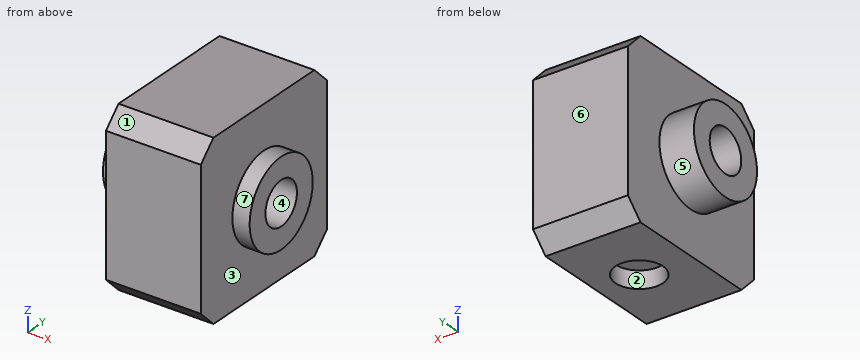
from build123d import *

# Parameters (mm, degrees)
SKETCH1_W           = 20
SKETCH1_H           = 20
BOSS_EXTRUDE1_DEPTH = 17
SKETCH2_R           = 15.353568197
SKETCH2_R_2         = 5
CUT_EXTRUDE1_DEPTH  = 2
CUT_EXTRUDE2_START  = -4
SKETCH3_R           = 15.635411304
SKETCH3_R_2         = 5
CUT_EXTRUDE2_DEPTH  = 4
SKETCH4_R           = 2.5
CUT_EXTRUDE3_DEPTH  = 23.113344387
CHAMFER1_SIZE       = 2
SKETCH5_R           = 2.75
CUT_EXTRUDE4_DEPTH  = 2


with BuildPart() as part:
    # Sketch1 → Boss-Extrude1 (new body)
    with BuildSketch(Plane(origin=(0, 0, 0), x_dir=(0, 0, -1), z_dir=(1, 0, 0))):
        Rectangle(SKETCH1_W, SKETCH1_H)
    extrude(amount=-BOSS_EXTRUDE1_DEPTH)

    # Sketch2 → Cut-Extrude1 (cut)
    with BuildSketch(Plane(origin=(0, 0, 0), x_dir=(0, 0, -1), z_dir=(1, 0, 0))):
        Circle(SKETCH2_R)
        Circle(SKETCH2_R_2, mode=Mode.SUBTRACT)
    extrude(amount=-CUT_EXTRUDE1_DEPTH, mode=Mode.SUBTRACT)

    # Sketch3 → Cut-Extrude2 (cut)
    with BuildSketch(Plane.ZY.offset(17).offset(CUT_EXTRUDE2_START)):
        Circle(SKETCH3_R)
        with Locations(Location((0, 0, 0), (0, 0, 180))):
            Circle(SKETCH3_R_2, mode=Mode.SUBTRACT)
    extrude(amount=CUT_EXTRUDE2_DEPTH, mode=Mode.SUBTRACT)

    # Sketch4 → Cut-Extrude3 (cut, through all)
    with BuildSketch(Plane(origin=(0, 0, 0), x_dir=(0, 0, -1), z_dir=(1, 0, 0))):
        Circle(SKETCH4_R)
    extrude(amount=-CUT_EXTRUDE3_DEPTH, mode=Mode.SUBTRACT)

    # Chamfer1
    chamfer1_edges = [part.edges().sort_by_distance(p)[0] for p in [
        (-7.5, -10, -10),
        (-7.5, -10, 10),
        (-7.5, 10, -10),
        (-7.5, 10, 10),
    ]]
    chamfer(chamfer1_edges, length=CHAMFER1_SIZE)

    # Sketch5 → Cut-Extrude4 (cut)
    with BuildSketch(Plane(origin=(0, 0, -10), x_dir=(-1, 0, 0), z_dir=(0, 0, -1))):
        with Locations(Location((7, 0, 0), (0, 0, 90))):
            Circle(SKETCH5_R)
    extrude(amount=-CUT_EXTRUDE4_DEPTH, mode=Mode.SUBTRACT)


solid = part.part
Work out the finished part from the listing and answer in its coordinate system (mm). Face numbers are marked on the shaded views. A direction names the side the tool comes from. Round coordinates to 2 decimals unless told otherwise and drop trailing zeros. Write each loop counter-clockwise with the first axis right and the second up, starting at its lowest first coordinate (ties: lowest second). Pieces come first, ordered by that corner, then holes. Notation, with made-up numbers: (30, 87) - (37, 87) arc R33 cw to (37, 121) - close; hole circle Ø7 at (38, -30). An arc over 180 degrees is marked (long way). Answer in a Markdown table with one row per item. Add a question column.
1. Find the intervals of material crossed by line 1 along Y through (x, z) = (-9.5, 0); line 2 along X through (y, z) = (0, -8.45); line 3 along Y through (x, z) = (-13.25, 0), in increasing order. Write a range as from..to.
2. The mould has two halves that part along Y. Classify the marked faces 1, 2, 3 and 4: +Y half, -Y half, draft (parallel to the pull), parting line (faces both ways), or undercut.
3. A cutting plane is placed at D-D, the plane y = -3.5. Determine the outline of the cut face in (x, z), and give its area (3 significant figures).
4. A cutting plane is placed at A-A, the plane x = -7. Determine the outline of the cut face in (y, z).
5. For the marked faces 5, 6 and 7, determine the directions among +Z, -Z, +X, -X, +Y, -Y from which every point of the face is accessible in a straight line to the end or side of a thin tool.
6. A cutting plane is placed at C-C, the plane z = 0. Determine the outline of the cut face in (x, y).
7. A cutting plane is placed at B-B, the plane y = 0. Determine the outline of the cut face in (x, z), and give its area (3 significant figures).
8. Given pin 1 (3 mm diameter, centred on x = -6.5, y = 0.5, fed in from -Z), flat-ended and moving along its own axis, determine where the tip first touches the part or whether it passes through.
Worked out:
| question | item | result |
|---|---|---|
| 1 | line 1 | -10..-2.5, 2.5..10 |
| 1 | line 2 | -13..-9.75, -4.25..-2 |
| 1 | line 3 | -5..-2.5, 2.5..5 |
| 2 | face 1 | -Y half |
| 2 | face 2 | undercut |
| 2 | face 3 | draft |
| 2 | face 4 | undercut |
| 3 | outline | (-17, -3.57) - (-13, -3.57) - (-13, -10) - (-2, -10) - (-2, -3.57) - (0, -3.57) - (0, 3.57) - (-2, 3.57) - (-2, 10) - (-13, 10) - (-13, 3.57) - (-17, 3.57) - close |
| 3 | area | 263 mm^2 |
| 4 | outline | (-10, -8) - (-8, -10) - (-2.75, -10) - (-2.75, -8) - (2.75, -8) - (2.75, -10) - (8, -10) - (10, -8) - (10, 8) - (8, 10) - (-8, 10) - (-10, 8) - close; hole circle Ø5 at (0, 0) |
| 5 | face 5 | -X |
| 5 | face 6 | +Z, -Z, +X, -X, +Y |
| 5 | face 7 | +X |
| 6 | outline | (-17, -5) - (-13, -5) - (-13, -10) - (-2, -10) - (-2, -5) - (0, -5) - (0, -2.5) - (-17, -2.5) - close; (-17, 2.5) - (0, 2.5) - (0, 5) - (-2, 5) - (-2, 10) - (-13, 10) - (-13, 5) - (-17, 5) - close |
| 7 | outline | (-17, -5) - (-13, -5) - (-13, -10) - (-9.75, -10) - (-9.75, -8) - (-4.25, -8) - (-4.25, -10) - (-2, -10) - (-2, -5) - (0, -5) - (0, -2.5) - (-17, -2.5) - close; (-17, 2.5) - (0, 2.5) - (0, 5) - (-2, 5) - (-2, 10) - (-13, 10) - (-13, 5) - (-17, 5) - close |
| 7 | area | 184 mm^2 |
| 8 | pin 1 | z = -8 |
